Design review of the part built by this model. Coordinates are the model's own, in mm. A direction names the side the tool comes from. Round coordinates to 2 decimals unless told otherwise and drop trailing zeros. Loops run counter-clockwise (first coordinate to the right, second up) from the corner with the lowest first, then second, coordinate; pieces in that order, holes last. Notation, with made-up numbers: (-19, 54) -> (38, 54) arc R31 ccw to (38, 84) -> close; hole circle Ø9 at (-3.75, -26). An arc over 180 degrees is marked (long way). Answer as CSV lines item,"result". Start each with the question number.
```python
from build123d import *

# Parameters (mm, degrees)
SKETCH_1_W          = 10
SKETCH_1_H          = 40
SKETCH_1_W_2        = 8
SKETCH_1_H_2        = 38
EXTRUDE_1_DEPTH     = 300
SKETCH_3_R          = 1.5
CUT_EXTRUDE_2_DEPTH = 10


with BuildPart() as part:
    # 草图1 → 凸台-拉伸1 (new body)
    with BuildSketch(Plane.XY):
        with Locations((5, 20)):
            Rectangle(SKETCH_1_W, SKETCH_1_H)
        with Locations((5, 20)):
            Rectangle(SKETCH_1_W_2, SKETCH_1_H_2, mode=Mode.SUBTRACT)
    extrude(amount=EXTRUDE_1_DEPTH)

    # 草图3 → 切除-拉伸2 (cut)
    with BuildSketch(Plane(origin=(10, 0, 0), x_dir=(0, 0, -1), z_dir=(1, 0, 0))):
        with Locations((-278, 18.5)):
            Circle(SKETCH_3_R)
        with Locations((-262, 18.5)):
            Circle(SKETCH_3_R)
        with Locations((-262, 3.5)):
            Circle(SKETCH_3_R)
        with Locations((-278, 3.5)):
            Circle(SKETCH_3_R)
    extrude(amount=-CUT_EXTRUDE_2_DEPTH, mode=Mode.SUBTRACT)


solid = part.part
```
Q1. Machinability: for faces 1 (the flat face through (1, 20, 148)), 2 (the flat face through (0, 20, 148)), which of the approach directions +Z, -Z, +X, -X, +Y, -Y give a long, thin tool a straight path to every point of the face, cutting with its end or side? Answer none if there is none.
Q2. Mouldability with a two-part tool opening along Y and no side actions: class faces 3 (the flat face through (5, 40, 148)), 4 (the flat face through (9, 20, 148)), 5 (the flat face through (5, 0, 148)) as pulls with the +Y half, pulls with the -Y half, needs draft (parallel to the pull), parting line crosses it, or undercut.
Q3. Add section A-A, the plane y = 23. Give the boundary of the cut face in (x, z).
Q4. Add section C-C, the plane z = 143.5. Give the boundary of the cut face in (x, y), and give its area (3 significant figures).
Q5. To check wall thickness, follow probe 1 along X at (y, z) = (22.5, 133.5); probe 2 along Y at (x, z) = (1.5, 232). State the ranges of each line that lie inside material, in increasing order. Write a range as from..to.
Q6. Add section B-B, the plane x = 7.25. Give the boundary of the cut face in (y, z), and give its area (3 significant figures).
Worked answers:
1,face 1,"+Z, -Z"
1,face 2,"+Z, -Z, -X, +Y, -Y"
2,face 3,"pulls with the +Y half"
2,face 4,"undercut"
2,face 5,"pulls with the -Y half"
3,outline,"(0, 0) -> (1, 0) -> (1, 300) -> (0, 300) -> close; (9, 0) -> (10, 0) -> (10, 300) -> (9, 300) -> close"
4,outline,"(0, 0) -> (10, 0) -> (10, 40) -> (0, 40) -> close; hole (1, 1) -> (9, 1) -> (9, 39) -> (1, 39) -> close"
4,area,"96.0 mm^2"
5,probe 1,"x = 0..1, 9..10"
5,probe 2,"y = 0..1, 39..40"
6,outline,"(0, 0) -> (1, 0) -> (1, 300) -> (0, 300) -> close; (39, 0) -> (40, 0) -> (40, 300) -> (39, 300) -> close"
6,area,"600 mm^2"
